Work out the finished part from the listing and answer in its coordinate system (mm). Face numbers are marked on the shaded views. A direction names the side the tool comes from. Round coordinates to 2 decimals unless told otherwise and drop trailing zeros. Order: outer loops, then holes, each group sorted by start corner. A loop starts at its lowest first (then second) coordinate and runs counter-clockwise, first axis right, second up. Notation, with made-up numbers: (62.25, 77.25) -> (91.25, 77.25) arc R14 cw to (91.25, 103.25) -> close; hole circle Ø10 at (11, 30.25). An arc over 180 degrees is marked (long way). Use a Markdown table: item, result. Add a question column.
Item 1: A tool of negligible diameter and unlimited length cuts with its end or side. For the marked faces 5, 6 and 7, from which of +Z, -Z, +X, -X, +Y, -Y can it reach the whole face along a straight path? Write none if from no direction.
Item 2: A cutting plane is placed at A-A, the plane z = 54. Determine the outline of the cut face in (x, y), plus the area to 3 significant figures.
Item 3: Find the intervals of material crossed by L1, parallel to X at y = 289, z = 47.5; L2, parallel to Y at x = 30, z = 65; L3, parallel to X at y = 130, z = 167, in increasing order. Write a range as [from, to].
Item 4: Flat-ended cylindrical pins translate along their axes: P1, Ø8, axis at x = 104.5, z = 198, coming from the -Y side; P2, Ø8, axis at x = 124.5, z = 54.5, coming from the -Y side; P3, Ø3, axis at x = 265, y = -163, coming from the +Z side. Find the tip coordinate at first contact, or state that the pin passes through.
Item 5: A cutting plane is placed at B-B, the plane y = 134. Determine the outline of the cut face in (x, z).
Item 6: For a pull along Y with two mould halves and no side action, classify the marked faces 1, 2, 3 and 4 as +Y half, -Y half, draft (parallel to the pull), parting line (faces both ways), or undercut.
Item 7: A cutting plane is placed at D-D, the plane x = 193.5. Determine the outline of the cut face in (y, z).
Item 8: A cutting plane is placed at C-C, the plane z = 121. Determine the outline of the cut face in (x, y).
from build123d import *

# Parameters (mm, degrees)
F0_W     = 387.35
F0_H     = 400.05
F1_DEPTH = 96.774
F2_T     = -1.27
F4_DEPTH = 400.05
F6_DEPTH = 387.35


with BuildPart() as f1:
    # F0 (on Top) → F1 (new body)
    with BuildSketch(Plane.XY):
        with Locations((92.767464, 103.439062)):
            Rectangle(F0_W, F0_H)
    extrude(amount=F1_DEPTH)

    # F2
    f2_openings = [f1.faces().sort_by_distance(p)[0] for p in [
        (92.767464, 103.439062, 96.774),
    ]]
    offset(amount=F2_T, openings=f2_openings)

    # F3 (on face) → F4 (join)
    with BuildSketch(Plane.XZ.offset(96.585938)):
        Polygon((-100.907536, 95.116133), (-100.907536, 96.774), (-256.567766, 227.388442), (-257.384107, 226.415566), align=None)
        Polygon((442.102695, 227.388442), (286.442464, 96.774), (286.442464, 95.116133), (442.919036, 226.415566), align=None)
    extrude(amount=-F4_DEPTH)

    # F5 (on face) → F6 (join)
    with BuildSketch(Plane.YZ.offset(286.442464)):
        Polygon((303.464062, 96.774), (303.464062, 95.116133), (437.3699, 207.476472), (436.553559, 208.449348), align=None)
        Polygon((-230.491776, 207.476472), (-96.585938, 95.116133), (-96.585938, 96.774), (-229.675435, 208.449348), align=None)
    extrude(amount=-F6_DEPTH)


solid = f1.part
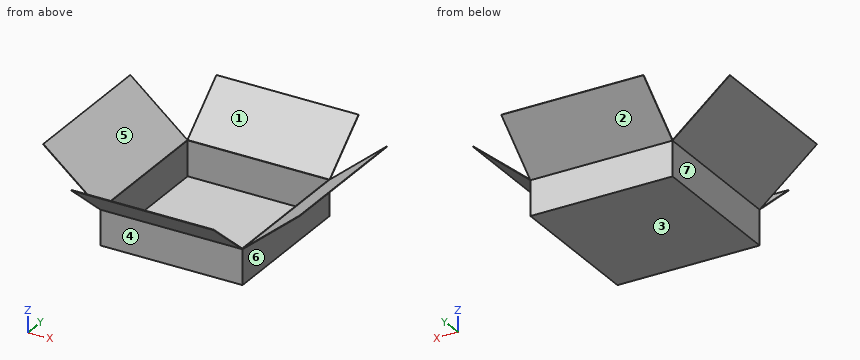
Reported:
| question | item | result |
|---|---|---|
| 1 | face 5 | +Z, +Y, -Y |
| 1 | face 6 | -Z, +X, +Y, -Y |
| 1 | face 7 | -Z, -X, +Y, -Y |
| 2 | outline | (-100.91, -96.59) -> (286.44, -96.59) -> (286.44, 303.46) -> (-100.91, 303.46) -> close; hole (-99.64, -95.32) -> (285.17, -95.32) -> (285.17, 302.19) -> (-99.64, 302.19) -> close |
| 2 | area | 1,990 mm² |
| 3 | L1 | [-100.91, -99.64], [285.17, 286.44] |
| 3 | L2 | [-96.59, -95.32], [302.19, 303.46] |
| 3 | L3 | [-186.58, -184.6], [370.13, 372.11] |
| 4 | P1 | y = -223.97 |
| 4 | P2 | y = -96.59 |
| 4 | P3 | z = 153.76 |
| 5 | outline | (-257.38, 226.42) -> (-100.91, 95.12) -> (-100.91, 0) -> (286.44, 0) -> (286.44, 95.12) -> (442.92, 226.42) -> (442.1, 227.39) -> (286.44, 96.77) -> (285.17, 96.77) -> (285.17, 1.27) -> (-99.64, 1.27) -> (-99.64, 96.77) -> (-100.91, 96.77) -> (-256.57, 227.39) -> close |
| 6 | face 1 | undercut |
| 6 | face 2 | +Y half |
| 6 | face 3 | draft |
| 6 | face 4 | -Y half |
| 7 | outline | (-230.49, 207.48) -> (-96.59, 95.12) -> (-96.59, 0) -> (303.46, 0) -> (303.46, 95.12) -> (437.37, 207.48) -> (436.55, 208.45) -> (303.46, 96.77) -> (302.19, 96.77) -> (302.19, 1.27) -> (-95.32, 1.27) -> (-95.32, 96.77) -> (-96.59, 96.77) -> (-229.68, 208.45) -> close |
| 8 | outline | (-131.75, -96.59) -> (-129.78, -96.59) -> (-129.78, 303.46) -> (-131.75, 303.46) -> close; (-100.91, -127.43) -> (286.44, -127.43) -> (286.44, -125.46) -> (-100.91, -125.46) -> close; (-100.91, 332.34) -> (286.44, 332.34) -> (286.44, 334.31) -> (-100.91, 334.31) -> close; (315.31, -96.59) -> (317.29, -96.59) -> (317.29, 303.46) -> (315.31, 303.46) -> close |
